from build123d import *

# Parameters (mm, degrees)
SKETCH1_R           = 2.3114
BOSS_EXTRUDE1_DEPTH = 12.7
SKETCH2_R           = 2.3114
CUT_EXTRUDE1_DEPTH  = 12.7
SKETCH6_W           = 14.121517248
SKETCH6_H           = 29.833964346
CUT_EXTRUDE2_DEPTH  = 12.7
SKETCH7_W           = 28.687814756
SKETCH7_H           = 15.668419498
CUT_EXTRUDE3_DEPTH  = 12.7


with BuildPart() as part:
    # Sketch1 → Boss-Extrude1 (new body)
    with BuildSketch(Plane(origin=(0, 0, 287.67498399), x_dir=(-1, 0, 0), z_dir=(0, 0, -1))):
        with BuildLine():
            Line((-152.251778141, 257.179185564), (-150.258610496, 257.179185564))
            Line((-150.258610496, 257.179185564), (-150.258610494, 278.616785564))
            ThreePointArc((-150.258610494, 278.616785564), (-149.678330448, 280.017705521), (-148.277410491, 280.597985567))
            Line((-148.277410491, 280.597985567), (-136.390210491, 280.597985564))
            Line((-136.390210491, 280.597985564), (-136.390210491, 279.429585564))
            Line((-136.390210491, 279.429585564), (-148.277410491, 279.429585567))
            ThreePointArc((-148.277410491, 279.429585567), (-148.852146887, 279.19152196), (-149.090210496, 278.616785564))
            Line((-149.090210496, 278.616785564), (-149.090210494, 277.111994182))
            Line((-149.090210494, 277.111994182), (-129.232034093, 277.111994182))
            Line((-129.232034093, 277.111994182), (-129.232034093, 316.653648997))
            ThreePointArc((-129.232034093, 316.653648997), (-134.566034093, 321.987648997), (-139.900034093, 316.653648997))
            Line((-139.900034093, 316.653648997), (-139.900034093, 289.375013802))
            ThreePointArc((-139.900034093, 289.375013802), (-144.05701735, 285.950698605), (-148.277410489, 282.604846529))
            ThreePointArc((-148.277410489, 282.604846529), (-151.211817414, 281.317505148), (-152.251778141, 278.286585564))
            Line((-152.251778141, 278.286585564), (-152.251778141, 257.179185564))
        make_face()
        with Locations((-134.383610491, 313.727499576)):
            Circle(SKETCH1_R, mode=Mode.SUBTRACT)
    extrude(amount=BOSS_EXTRUDE1_DEPTH)

    # Sketch2 → Cut-Extrude1 (cut)
    with BuildSketch(Plane.ZY.offset(-150.25861052)):
        with Locations((281.230197131, 274.312688508)):
            Circle(SKETCH2_R)
        with Locations((281.230197131, 261.612688508)):
            Circle(SKETCH2_R)
    extrude(amount=-CUT_EXTRUDE1_DEPTH, mode=Mode.SUBTRACT)

    # Sketch5 → CBORE for #8 Button Head Cap Screw1 (revolve, cut)
    with BuildSketch(Plane(origin=(142.708000895, 290.757985564, 281.067357509), x_dir=(0, 0, 1), z_dir=(1, 0, 0))):
        Polygon((0, 0), (0, 33.5788), (2.2479, 33.5788), (2.2479, 7.2898), (4.36626, 7.2898), (4.36626, 0), align=None)
    revolve(axis=Axis((142.708000895, 297.107985564, 281.067357509), (0, -1, 0)), mode=Mode.SUBTRACT)

    # Sketch6 → Cut-Extrude2 (cut)
    with BuildSketch(Plane(origin=(0, 0, 274.97498399), x_dir=(-1, 0, 0), z_dir=(0, 0, -1))):
        with Locations((-155.338169113, 267.687864356)):
            Rectangle(SKETCH6_W, SKETCH6_H)
    extrude(amount=-CUT_EXTRUDE2_DEPTH, mode=Mode.SUBTRACT)

    # Sketch7 → Cut-Extrude3 (cut)
    with BuildSketch(Plane(origin=(0, 0, 274.97498399), x_dir=(-1, 0, 0), z_dir=(0, 0, -1))):
        with Locations((-133.933503111, 272.763775818)):
            Rectangle(SKETCH7_W, SKETCH7_H)
    extrude(amount=-CUT_EXTRUDE3_DEPTH, mode=Mode.SUBTRACT)


solid = part.part
Check sheet for the modelled part. Datum: model origin and axes. Units: mm. A direction names the side the tool comes from. Round coordinates to 2 decimals unless told otherwise and drop trailing zeros. Loops run counter-clockwise (first coordinate to the right, second up) from the corner with the lowest first, then second, coordinate; pieces in that order, holes last.
1. Set-up check for faces 4 (the flat face through (129.232, 298, 281)), 5 (the flat face through (145, 283.468, 279)): record each of +Z, -Z, +X, -X, +Y, -Y from which the full face is reachable in a straight line by a thin tool's end or side.
2. Sectioned sample at B-B on x = 135.25. Record the boundary of the cut face in (y, z), and give its area (3 significant figures).
3. Sectioned sample at A-A on z = 282. Record the boundary of the cut face in (x, y), and give its area (3 significant figures).
4. Sectioned sample at D-D on z = 276. Record the boundary of the cut face in (x, y).
5. Mould release check, pull along X, two halves, no side actions. Record for faces 1 (the flat face through (139, 290.758, 281)), 2 (the cylindrical face through (143.569, 282.053, 283.144)), 3 (the flat face through (139.9, 303, 281)): released by +X, released by -X, zero draft, split by the parting line, or undercut.
6. Scan lines: probe 1 along Y at (x, z) = (135.5, 276.25); probe 2 along Y at (x, z) = (133.5, 280); probe 3 along X at (y, z) = (295.5, 282.5). Record each from-to range of solid material in increasing order.
7. Gauge pin test, flat ends, axial feed: pin 1 Ø7.5 at (x, y) = (134.38, 313.73) entering from -Z (3 decimals); pin 2 Ø5 at (x, z) = (142.71, 281.07) entering from +Y; pin 3 Ø2.5 at (x, z) = (142.71, 281.07) entering from -Y. Record the tip position at first contact, or that the pin passes through.
8. Sectioned sample at C-C on y = 313. Record the boundary of the cut face in (x, z).
Recorded:
1. face 4: +Z, -Z, -X, +Y, -Y
1. face 5: none
2. outline: (280.6, 274.97) - (311.58, 274.97) - (311.58, 287.67) - (280.6, 287.67) - close; (315.87, 274.97) - (321.94, 274.97) - (321.94, 287.67) - (315.87, 287.67) - close
2. area: 471 mm2
3. outline: (129.23, 280.6) - (140.66, 280.6) - (140.66, 283.47) - (138.44, 283.47) - (138.44, 290.76) - (139.9, 290.76) - (139.9, 316.65) arc R5.33 ccw to (129.23, 316.65) - close; (144.75, 280.6) - (148.28, 280.6) - (148.28, 282.6) arc R287.53 cw to (146.97, 283.62) - (146.97, 283.47) - (144.75, 283.47) - close; hole circle Ø4.62 at (134.38, 313.73)
3. area: 414 mm2
4. outline: (129.23, 280.6) - (148.28, 280.6) - (148.28, 282.6) arc R287.53 cw to (139.9, 289.38) - (139.9, 316.65) arc R5.33 ccw to (129.23, 316.65) - close; hole circle Ø4.62 at (134.38, 313.73)
5. face 1: zero draft
5. face 2: undercut
5. face 3: released by +X
6. probe 1: y = 280.6 to 311.7, 315.75 to 321.91
6. probe 2: y = 280.6 to 311.59, 315.86 to 321.88
6. probe 3: x = 129.23 to 139.9
7. pin 1: stops at z = 274.975
7. pin 2: stops at y = 283.47
7. pin 3: passes through
8. outline: (129.23, 274.97) - (132.19, 274.97) - (132.19, 287.67) - (129.23, 287.67) - close; (136.58, 274.97) - (139.9, 274.97) - (139.9, 287.67) - (136.58, 287.67) - close
